Autodesk Fusion 360 part; units mm, degrees
sketch "Sketch1" plane through (0, 0, 0) normal (0, 0, 1) x (1, 0, 0)
  circle A0 centre (0, 0) radius 23.75
  line L0 (49.96, 2) -> (39.96, 2)
  line L1 (39.96, 2) -> (39.96, -2)
  line L2 (39.96, -2) -> (49.96, -2)
  line L3 (44.1446, 23.4788) -> (35.1349, 19.1399)
  line L4 (36.8705, 15.536) -> (45.8802, 19.8749)
  line L5 (35.1349, 19.1399) -> (36.8705, 15.536)
  line L6 (29.5859, 40.3073) -> (23.351, 32.489)
  line L7 (26.4783, 29.995) -> (32.7132, 37.8133)
  line L8 (23.351, 32.489) -> (26.4783, 29.995)
  line L9 (9.1673, 49.1524) -> (6.9421, 39.4031)
  line L10 (10.8418, 38.5131) -> (13.067, 48.2623)
  line L11 (6.9421, 39.4031) -> (10.8418, 38.5131)
  line L12 (-13.067, 48.2623) -> (-10.8418, 38.5131)
  line L13 (-6.9421, 39.4031) -> (-9.1673, 49.1524)
  line L14 (-10.8418, 38.5131) -> (-6.9421, 39.4031)
  line L15 (-32.7132, 37.8133) -> (-26.4783, 29.995)
  line L16 (-23.351, 32.489) -> (-29.5859, 40.3073)
  line L17 (-26.4783, 29.995) -> (-23.351, 32.489)
  line L18 (-45.8802, 19.8749) -> (-36.8705, 15.536)
  line L19 (-35.1349, 19.1399) -> (-44.1446, 23.4788)
  line L20 (-36.8705, 15.536) -> (-35.1349, 19.1399)
  line L21 (-49.96, -2) -> (-39.96, -2)
  line L22 (-39.96, 2) -> (-49.96, 2)
  line L23 (-39.96, -2) -> (-39.96, 2)
  line L24 (-44.1446, -23.4788) -> (-35.1349, -19.1399)
  line L25 (-36.8705, -15.536) -> (-45.8802, -19.8749)
  line L26 (-35.1349, -19.1399) -> (-36.8705, -15.536)
  line L27 (-29.5859, -40.3073) -> (-23.351, -32.489)
  line L28 (-26.4783, -29.995) -> (-32.7132, -37.8133)
  line L29 (-23.351, -32.489) -> (-26.4783, -29.995)
  line L30 (-9.1673, -49.1524) -> (-6.9421, -39.4031)
  line L31 (-10.8418, -38.5131) -> (-13.067, -48.2623)
  line L32 (-6.9421, -39.4031) -> (-10.8418, -38.5131)
  line L33 (13.067, -48.2623) -> (10.8418, -38.5131)
  line L34 (6.9421, -39.4031) -> (9.1673, -49.1524)
  line L35 (10.8418, -38.5131) -> (6.9421, -39.4031)
  line L36 (32.7132, -37.8133) -> (26.4783, -29.995)
  line L37 (23.351, -32.489) -> (29.5859, -40.3073)
  line L38 (26.4783, -29.995) -> (23.351, -32.489)
  line L39 (45.8802, -19.8749) -> (36.8705, -15.536)
  line L40 (35.1349, -19.1399) -> (44.1446, -23.4788)
  line L41 (36.8705, -15.536) -> (35.1349, -19.1399)
  arc A1 (49.96, 2) -> (45.8802, 19.8749) centre (0, 0) ccw
  arc A2 (44.1446, 23.4788) -> (32.7132, 37.8133) centre (0, 0) ccw
  arc A3 (29.5859, 40.3073) -> (13.067, 48.2623) centre (0, 0) ccw
  arc A4 (9.1673, 49.1524) -> (-9.1673, 49.1524) centre (0, 0) ccw
  arc A5 (-13.067, 48.2623) -> (-29.5859, 40.3073) centre (0, 0) ccw
  arc A6 (-32.7132, 37.8133) -> (-44.1446, 23.4788) centre (0, 0) ccw
  arc A7 (-45.8802, 19.8749) -> (-49.96, 2) centre (0, 0) ccw
  arc A8 (-49.96, -2) -> (-45.8802, -19.8749) centre (0, 0) ccw
  arc A9 (-44.1446, -23.4788) -> (-32.7132, -37.8133) centre (0, 0) ccw
  arc A10 (-29.5859, -40.3073) -> (-13.067, -48.2623) centre (0, 0) ccw
  arc A11 (-9.1673, -49.1524) -> (9.1673, -49.1524) centre (0, 0) ccw
  arc A12 (13.067, -48.2623) -> (29.5859, -40.3073) centre (0, 0) ccw
  arc A13 (32.7132, -37.8133) -> (44.1446, -23.4788) centre (0, 0) ccw
  arc A14 (45.8802, -19.8749) -> (49.96, -2) centre (0, 0) ccw
  dimension "d1" = 100
  dimension "d6" = 47.5
  dimension "d7" = 10
  dimension "d8" = 10
  dimension "d9" = 4
  dimension "d11" = 360
extrude "Extrude1" add sketch "Sketch1" along normal blind 4
equation "d1 = D_o"
equation "D_o = 100 mm"
equation "D_i = 47.5 mm"
equation "offset = 10 mm"
equation "d6 = D_i"
equation "d7 = offset"
equation "d8 = offset"
equation "d9 = Linear Dimension-4"
The listing builds one solid part. Answer for the finished solid, in the listing's coordinates (mm). A direction names the side the tool comes from. Give positions to 0.01 mm unless a question says otherwise; leave off trailing zeros. Order: outer loops, then holes, each group sorted by start corner. A loop starts at its lowest first (then second) coordinate and runs counter-clockwise, first axis right, second up.
Item 1: Given pin 1 Ø1.2 at (y, z) = (0.5, 2.5) entering from +X; pin 2 Ø1.2 at (x, z) = (-46, 2.5) entering from -Y; pin 3 Ø1.2 at (y, z) = (-1, 1.5) entering from -X, each flat-ended and moving along its own axis, determine where each tip first touches the part or whether it passes through.
From the geometry:
pin 1: stops at x = 39.96
pin 2: stops at y = -19.87
pin 3: stops at x = -39.96
Item 2: Find the intervals of material crossed by probe 1 along Y at (x, z) = (0, 0.9); probe 2 along Y at (x, z) = (-36, 2.7); probe 3 along Y at (x, z) = (28, 3.8), in increasing order.
From the geometry:
probe 1: y = -50 to -23.75, 23.75 to 50
probe 2: y = -34.7 to -19.56, -17.34 to 17.34, 19.56 to 34.7
probe 3: y = -41.42 to -38.32, -31.9 to 31.9, 38.32 to 41.42
Item 3: Which of the six approach directions +Z, -Z, +X, -X, +Y, -Y give full straight-line access (tool end or side, diameter ignored) to faces 4 (the face through (-11.94, -43.32, 1.97)), 5 (the face through (21.81, -44.992, 1.972)), 6 (the face through (26.51, 36.45, 1.97)), 7 (the face through (11.94, 43.32, 1.97)), 8 (the face through (-45, -2, 2))?
From the geometry:
face 4: +Z, -Z, -Y
face 5: +Z, -Z, +X, -Y
face 6: +Z, -Z
face 7: +Z, -Z, +Y
face 8: +Z, -Z, -X
Item 4: For a pull along Y with two mould halves and no side action, classify faces 1 (the face through (10, -22, 4)), 2 (the face through (39.011, 31.275, 1.972)), 3 (the face through (8.04, -44.21, 1.97)) as pulls with the +Y half, pulls with the -Y half, needs draft (parallel to the pull), parting line crosses it, or undercut.
From the geometry:
face 1: needs draft
face 2: pulls with the +Y half
face 3: undercut
Item 5: The part is cut by section A-A, the plane x = 0. Give the vertices of the cut face in (y, z).
From the geometry:
outline: (-50, 0) - (-23.75, 0) - (-23.75, 4) - (-50, 4) - close; (23.75, 0) - (50, 0) - (50, 4) - (23.75, 4) - close
Item 6: The part is cut by section B-B, the plane y = 0. Give the vertices of the cut face in (x, z).
From the geometry:
outline: (-39.96, 0) - (-23.75, 0) - (-23.75, 4) - (-39.96, 4) - close; (23.75, 0) - (39.96, 0) - (39.96, 4) - (23.75, 4) - close
